Design review of the part shown in the three views and the two pictorial views. Dimensions are in mm from the part's minimum x, y and z. A direction names the side the tool comes from. Coordinates: 2 decimals unless noted, no trailing zeros. Write each loop counter-clockwise with the first axis right and the second up, starting at its lowest first coordinate (ties: lowest second). Pieces come first, ordered by that corner, then holes. Notation, with made-up numbers: (78.25, 33.25) -> (109.25, 33.25) arc R25 ccw to (109.25, 49.25) -> close; hole circle Ø5 at (65.5, 87). An arc over 180 degrees is marked (long way). Answer in a Markdown table with one row per item. Add a question column.
Item 1: To check wall thickness, follow line 1 (X direction, y = 5, z = 4); line 2 (Z direction, x = 14, y = 4); line 3 (X direction, y = 5.75, z = 6.5). State the ranges of each line that lie inside material, in increasing order.
Item 2: Clearance check with flat-ended pins moving along their axes: P1, Ø1.5, axis at x = 18.5, y = 3, coming from the -Z side; P2, Ø3, axis at x = 13, y = 6, coming from the +Z side; P3, Ø1, axis at x = 19, z = 4, coming from the -Y side. State where each tip first meets the part, or that it passes through.
Item 3: Take a section at A-A, the plane z = 4. Write out the cut boundary in (x, y).
Item 4: Take a section at D-D, the plane x = 14. Write out the cut boundary in (y, z), and give its area (3 significant figures).
Item 5: For the marked faces 1 and 2, list the 3-axis set-ups (+Z, -Z, +X, -X, +Y, -Y) from which the entire face can be reached by the end or side of a thin tool; tool diameter is ignored.
Item 6: Take a section at B-B, the plane y = 4. Write out the cut boundary in (x, z).
Item 7: Take a section at C-C, the plane x = 7. Write out the cut boundary in (y, z).
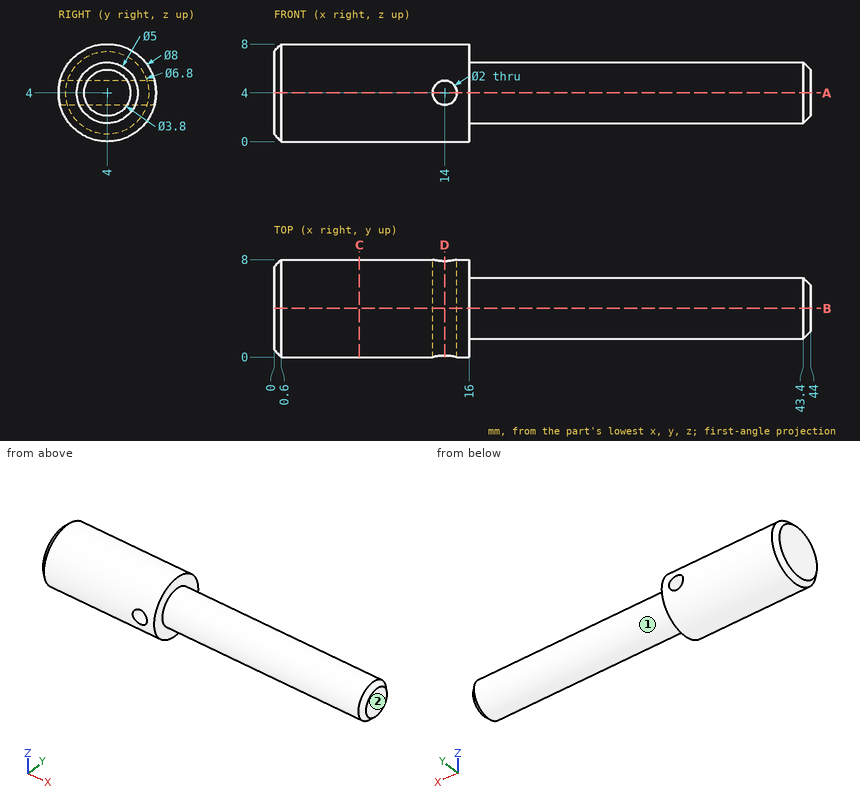
Answers:
| question | item | result |
|---|---|---|
| 1 | line 1 | x = 0 to 13, 15 to 44 |
| 1 | line 2 | z = 0 to 3, 5 to 8 |
| 1 | line 3 | x = 0 to 16 |
| 2 | P1 | stops at z = 1.51 |
| 2 | P2 | stops at z = 7.97 |
| 2 | P3 | stops at y = 1.5 |
| 3 | outline | (0, 0.6) -> (0.6, 0) -> (13, 0) -> (13, 8) -> (0.6, 8) -> (0, 7.4) -> close; (15, 0) -> (16, 0) -> (16, 1.5) -> (43.4, 1.5) -> (44, 2.1) -> (44, 5.9) -> (43.4, 6.5) -> (16, 6.5) -> (16, 8) -> (15, 8) -> close |
| 4 | outline | (0.13, 3) arc R4 ccw to (7.87, 3) -> close; (0.13, 5) -> (7.87, 5) arc R4 ccw to start |
| 4 | area | 34.4 mm^2 |
| 5 | face 1 | +X |
| 5 | face 2 | +Z, -Z, +X, +Y, -Y |
| 6 | outline | (0, 0.6) -> (0.6, 0) -> (16, 0) -> (16, 1.5) -> (43.4, 1.5) -> (44, 2.1) -> (44, 5.9) -> (43.4, 6.5) -> (16, 6.5) -> (16, 8) -> (0.6, 8) -> (0, 7.4) -> close; hole circle Ø2 at (14, 4) |
| 7 | outline | circle Ø8 at (4, 4) |
